Read the model definition and answer for the solid it produces. Units are mm, in the model's axes. Round coordinates to 2 decimals unless told otherwise and drop trailing zeros. Order: outer loops, then holes, each group sorted by start corner. A loop starts at its lowest first (then second) coordinate and runs counter-clockwise, first axis right, second up.
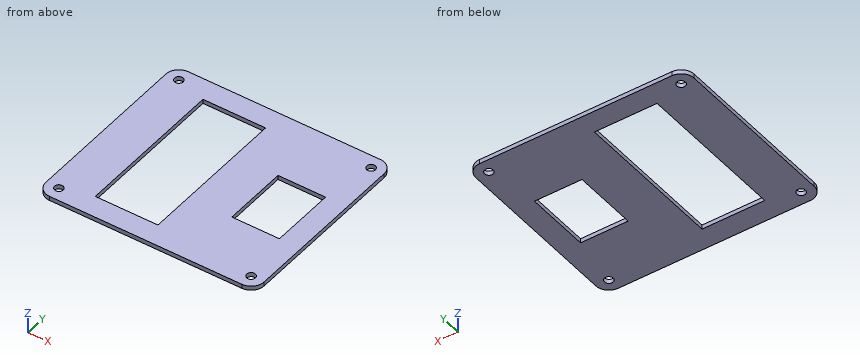
from build123d import *

# Parameters (mm, degrees)
F0_R     = 2
F0_W     = 29
F0_H     = 70
F0_W_2   = 22
F0_H_2   = 30
F1_DEPTH = 2


with BuildPart() as f1:
    # F0 (on Top) → F1 (new body)
    with BuildSketch(Plane.XY):
        with BuildLine():
            Line((-95, 0), (-6, 0))
            ThreePointArc((-6, 0), (-1.757359, 1.757359), (0, 6))
            Line((0, 6), (0, 84))
            ThreePointArc((0, 84), (-1.757359, 88.242641), (-6, 90))
            Line((-6, 90), (-95, 90))
            ThreePointArc((-95, 90), (-99.242641, 88.242641), (-101, 84))
            Line((-101, 84), (-101, 6))
            ThreePointArc((-101, 6), (-99.242641, 1.757359), (-95, 0))
        make_face()
        with Locations((-95, 6)):
            Circle(F0_R, mode=Mode.SUBTRACT)
        with Locations((-6, 6)):
            Circle(F0_R, mode=Mode.SUBTRACT)
        with Locations((-66.5, 45)):
            Rectangle(F0_W, F0_H, mode=Mode.SUBTRACT)
        with Locations((-95, 84)):
            Circle(F0_R, mode=Mode.SUBTRACT)
        with Locations((-21, 45)):
            Rectangle(F0_W_2, F0_H_2, mode=Mode.SUBTRACT)
        with Locations((-6, 84)):
            Circle(F0_R, mode=Mode.SUBTRACT)
    extrude(amount=F1_DEPTH)


solid = f1.part
Q1. A cutting plane is placed at A-A, the plane y = 50.5. Give the vertices of the cut face in (x, z).
Outcome:
outline: (-101, 0) - (-81, 0) - (-81, 2) - (-101, 2) - close; (-52, 0) - (-32, 0) - (-32, 2) - (-52, 2) - close; (-10, 0) - (0, 0) - (0, 2) - (-10, 2) - close
Q2. A cutting plane is placed at C-C, the plane y = 71.5. Give the vertices of the cut face in (x, z), plus the area to 3 significant figures.
Outcome:
outline: (-101, 0) - (-81, 0) - (-81, 2) - (-101, 2) - close; (-52, 0) - (0, 0) - (0, 2) - (-52, 2) - close
area: 144 mm2
Q3. A cutting plane is placed at D-D, the plane z = 1.25. Give the vertices of the cut face in (x, y).
Outcome:
outline: (-101, 6) arc R6 ccw to (-95, 0) - (-6, 0) arc R6 ccw to (0, 6) - (0, 84) arc R6 ccw to (-6, 90) - (-95, 90) arc R6 ccw to (-101, 84) - close; hole circle Ø4 at (-95, 6); hole circle Ø4 at (-95, 84); hole (-81, 10) - (-52, 10) - (-52, 80) - (-81, 80) - close; hole (-32, 30) - (-10, 30) - (-10, 60) - (-32, 60) - close; hole circle Ø4 at (-6, 6); hole circle Ø4 at (-6, 84)
Q4. Straight lines are drawn through the part: probe 1 along Y at (x, z) = (-95, 1.5); probe 2 along X at (y, z) = (48.5, 1); probe 3 along Y at (x, z) = (-70.5, 0.3). For each, find the intervals that lie inside material, in ascending order.
Outcome:
probe 1: y = 0 to 4, 8 to 82, 86 to 90
probe 2: x = -101 to -81, -52 to -32, -10 to 0
probe 3: y = 0 to 10, 80 to 90
Q5. A cutting plane is placed at B-B, the plane x = -68. Give the vertices of the cut face in (y, z).
Outcome:
outline: (0, 0) - (10, 0) - (10, 2) - (0, 2) - close; (80, 0) - (90, 0) - (90, 2) - (80, 2) - close
